Geometry: final body of the model. Coordinates: model frame, mm. A direction names the side the tool comes from. Round coordinates to 2 decimals unless told otherwise and drop trailing zeros. Loops run counter-clockwise (first coordinate to the right, second up) from the corner with the lowest first, then second, coordinate; pieces in that order, holes last. Notation, with made-up numbers: (-8, 10.5) - (22, 10.5) arc R11 ccw to (22, 24.5) - close; hole circle Ø8 at (86, 29). An arc over 180 degrees is marked (long way). Answer as CSV lines item,"result".
from build123d import *

# Parameters (mm, degrees)
ESQUISSE1_R             = 31
BOSS_EXTRU_1_DEPTH      = 14
ESQUISSE2_R             = 22.5
ESQUISSE2_R_2           = 12.5
ENL_V_MAT_EXTRU_1_DEPTH = 3


with BuildPart() as part:
    # Esquisse1 → Boss.-Extru.1 (new body)
    with BuildSketch(Plane.XY):
        Circle(ESQUISSE1_R)
    extrude(amount=BOSS_EXTRU_1_DEPTH)

    # Esquisse2 → Enlèv. mat.-Extru.1 (cut)
    with BuildSketch(Plane(origin=(0, 0, 0), x_dir=(-1, 0, 0), z_dir=(0, 0, -1))):
        Circle(ESQUISSE2_R)
        Circle(ESQUISSE2_R_2, mode=Mode.SUBTRACT)
    extrude(amount=-ENL_V_MAT_EXTRU_1_DEPTH, mode=Mode.SUBTRACT)


solid = part.part
(1) Access query for faces 1 (the face through (-10, -10, 3)), 2 (the face through (21, 9, 0)). Directions: +Z, -Z, +X, -X, +Y, -Y. A direction counts if a zero-diameter tool reaches every point of the face in a straight line with its end or side. Return the directions, or none.
Findings below:
face 1,"-Z"
face 2,"-Z, +X, -X, +Y, -Y"
(2) Draft query along Y for faces 3 (the face through (-4.036, 30.736, 6.902)), 4 (the face through (-11.923, 3.755, 1.479)), 5 (the face through (0, 0, 0)). Return one class per face: pulls with the +Y half, pulls with the -Y half, needs draft (parallel to the pull), parting line crosses it, or undercut.
Findings below:
face 3,"parting line crosses it"
face 4,"undercut"
face 5,"needs draft"
(3) Section B-B (x = 0). Output: boundary loops of the cut face in (y, z).
Findings below:
outline,"(-31, 0) - (-22.5, 0) - (-22.5, 3) - (-12.5, 3) - (-12.5, 0) - (12.5, 0) - (12.5, 3) - (22.5, 3) - (22.5, 0) - (31, 0) - (31, 14) - (-31, 14) - close"
(4) Material intervals for line 1 along Y through (x, z) = (0, 0.7); line 2 along Y through (x, z) = (-3, 2.25); line 3 along X through (y, z) = (1, 9.5), sorted ascending.
Findings below:
line 1,"-31 to -22.5, -12.5 to 12.5, 22.5 to 31"
line 2,"-30.85 to -22.3, -12.13 to 12.13, 22.3 to 30.85"
line 3,"-30.98 to 30.98"
(5) Section D-D (z = 5.75). Output: boundary loops of the cut face in (x, y), and give its area (3 significant figures).
Findings below:
outline,"circle Ø62 at (0, 0)"
area,"3,020 mm2"
(6) Section A-A (z = 1.25). Output: boundary loops of the cut face in (x, y).
Findings below:
outline,"circle Ø62 at (0, 0); circle Ø25 at (0, 0); hole circle Ø45 at (0, 0)"
(7) Pin query (flat end, axial travel): P1, Ø4, axis at y = -20, z = 2.5, coming from the -X side; P2, Ø1, axis at x = 24, z = 10.5, coming from the -Y side; P3, Ø2, axis at y = 6.5, z = 5.5, coming from the -X side. Return the tip coordinate at first contact, or that it passes through.
Findings below:
P1,"x = -25.24"
P2,"y = -20.22"
P3,"x = -30.51"
